```python
from build123d import *

# Parameters (mm, degrees)
SKETCH1_R               = 150
BOSS_EXTRUDE1_DEPTH     = 100
FILLET1_R               = 25
CUT_EXTRUDE1_DEPTH      = 300
CUT_EXTRUDE1_DEPTH_BACK = 300
CUT_EXTRUDE2_DEPTH      = 300
CUT_EXTRUDE2_DEPTH_BACK = 300
SKETCH5_R               = 25


with BuildPart() as part:
    # Sketch1 → Boss-Extrude1 (new body)
    with BuildSketch(Plane.XY):
        Circle(SKETCH1_R)
    extrude(amount=BOSS_EXTRUDE1_DEPTH)

    # Fillet1
    fillet1_edges = [part.edges().sort_by_distance(p)[0] for p in [
        (-150, 0, 0),
        (-150, 0, 100),
    ]]
    fillet(fillet1_edges, radius=FILLET1_R)

    # Sketch4 → Cut-Extrude1 (cut, two sides: drawn at the far end of the back side and taken through both)
    with BuildSketch(Plane.XY.offset(-CUT_EXTRUDE1_DEPTH_BACK)):
        with BuildLine():
            Line((82.731493399, 82.731493399), (21.920310217, 21.920310217))
            ThreePointArc((21.920310217, 21.920310217), (25.775557981, 17.222677224), (28.640265508, 11.863186403))
            Line((28.640265508, 11.863186403), (108.093905304, 44.773961587))
            ThreePointArc((108.093905304, 44.773961587), (97.281944639, 65.001717263), (82.731493399, 82.731493399))
        make_face()
        with BuildLine():
            Line((0, 117), (0, 31))
            ThreePointArc((0, 31), (6.047799982, 30.404343693), (11.863186403, 28.640265508))
            Line((11.863186403, 28.640265508), (44.773961587, 108.093905304))
            ThreePointArc((44.773961587, 108.093905304), (22.825567676, 114.751877807), (0, 117))
        make_face()
        with BuildLine():
            Line((-82.731493399, 82.731493399), (-21.920310217, 21.920310217))
            ThreePointArc((-21.920310217, 21.920310217), (-17.222677224, 25.775557981), (-11.863186403, 28.640265508))
            Line((-11.863186403, 28.640265508), (-44.773961587, 108.093905304))
            ThreePointArc((-44.773961587, 108.093905304), (-65.001717263, 97.281944639), (-82.731493399, 82.731493399))
        make_face()
        with BuildLine():
            Line((-117, 0), (-31, 0))
            ThreePointArc((-31, 0), (-30.404343693, 6.047799983), (-28.640265508, 11.863186403))
            Line((-28.640265508, 11.863186403), (-108.093905304, 44.773961587))
            ThreePointArc((-108.093905304, 44.773961587), (-114.751877807, 22.825567676), (-117, 0))
        make_face()
        with BuildLine():
            Line((-82.731493399, -82.731493399), (-21.920310217, -21.920310217))
            ThreePointArc((-21.920310217, -21.920310217), (-25.775557981, -17.222677224), (-28.640265508, -11.863186403))
            Line((-28.640265508, -11.863186403), (-108.093905304, -44.773961587))
            ThreePointArc((-108.093905304, -44.773961587), (-97.281944639, -65.001717263), (-82.731493399, -82.731493399))
        make_face()
        with BuildLine():
            Line((0, -117), (0, -31))
            ThreePointArc((0, -31), (-6.047799983, -30.404343693), (-11.863186403, -28.640265508))
            Line((-11.863186403, -28.640265508), (-44.773961587, -108.093905304))
            ThreePointArc((-44.773961587, -108.093905304), (-22.825567676, -114.751877807), (0, -117))
        make_face()
        with BuildLine():
            Line((82.731493399, -82.731493399), (21.920310217, -21.920310217))
            ThreePointArc((21.920310217, -21.920310217), (17.222677224, -25.775557981), (11.863186403, -28.640265508))
            Line((11.863186403, -28.640265508), (44.773961587, -108.093905304))
            ThreePointArc((44.773961587, -108.093905304), (65.001717263, -97.281944639), (82.731493399, -82.731493399))
        make_face()
        with BuildLine():
            Line((117, 0), (31, 0))
            ThreePointArc((31, 0), (30.404343693, -6.047799983), (28.640265508, -11.863186403))
            Line((28.640265508, -11.863186403), (108.093905304, -44.773961587))
            ThreePointArc((108.093905304, -44.773961587), (114.751877807, -22.825567676), (117, 0))
        make_face()
    extrude(amount=CUT_EXTRUDE1_DEPTH + CUT_EXTRUDE1_DEPTH_BACK, mode=Mode.SUBTRACT)

    # Sketch5 → Cut-Extrude2 (cut, two sides: drawn at the far end of the back side and taken through both)
    with BuildSketch(Plane.XY.offset(-CUT_EXTRUDE2_DEPTH_BACK)):
        Circle(SKETCH5_R)
    extrude(amount=CUT_EXTRUDE2_DEPTH + CUT_EXTRUDE2_DEPTH_BACK, mode=Mode.SUBTRACT)


solid = part.part
```
The model under review builds one solid part; all positions refer to its coordinate system, in mm. Round coordinates to 2 decimals unless told otherwise and drop trailing zeros. Write item = value, one per line.
Item 1: For line 1 (X direction, y = -90, z = 93.5); line 2 (X direction, y = 21.5, z = 75.5); line 3 (Y direction, x = 39.5, z = 32), list the stretches that pass through material, from the lowest coordinate up. Write a range as [from, to].
Return value:
line_1 = [-109.6, -37.28], [0, 37.28], [74.76, 109.6]
line_2 = [-148.45, -115.01], [-51.91, -12.76], [12.76, 22.33], [51.91, 148.45]
line_3 = [-144.71, -95.36], [-39.5, -16.36], [0, 16.36], [39.5, 95.36], [110.13, 144.71]
Item 2: The part is to be moulded in two halves that separate along Y. For faces 1 (the cylindrical face through (-19.527, 148.724, 49.65)), 2 (the flat face through (26, 2, 100)), 3 (the flat face through (53, -53, 49)), 4 (the cylindrical face through (114.69, -23.14, 49.3)), say which applies: released by +Y, released by -Y, zero draft, split by the parting line, or undercut.
Return value:
face_1 = split by the parting line
face_2 = zero draft
face_3 = undercut
face_4 = undercut
Item 3: Take a section at A-A on z = 47. State how many separate pieces and enclosed holes the cut face has, then the cut area to 3 significant figures.
Return value:
separate_pieces = 1
enclosed_holes = 9
area = 48,700 mm2
Item 4: Insertion check: P1, Ø3, axis at x = -104.5, z = 48.5, coming from the -Y side; P2, Ø1.5, axis at y = 5, z = 72.5, coming from the -X side; P3, Ø3, axis at x = 11.5, z = 90, coming from the +Y side. Each pin has a flat end and moves straight along its axis. Give the tip position at first contact, or say it passes through.
Return value:
P1 = -109.05
P2 = -149.94
P3 = 145.6
